Design review of the part built by this model. Coordinates are the model's own, in mm. Coordinates: 2 decimals unless noted, no trailing zeros. Order: outer loops, then holes, each group sorted by start corner. A loop starts at its lowest first (then second) coordinate and runs counter-clockwise, first axis right, second up. Notation, with made-up numbers: (11, -18) - (43, -18) arc R22 cw to (43, 15) - close; hole circle Ø2 at (66.5, 35). An arc over 180 degrees is marked (long way). Write each question's results on one line, items separated by ' | '. Start each with the question number.
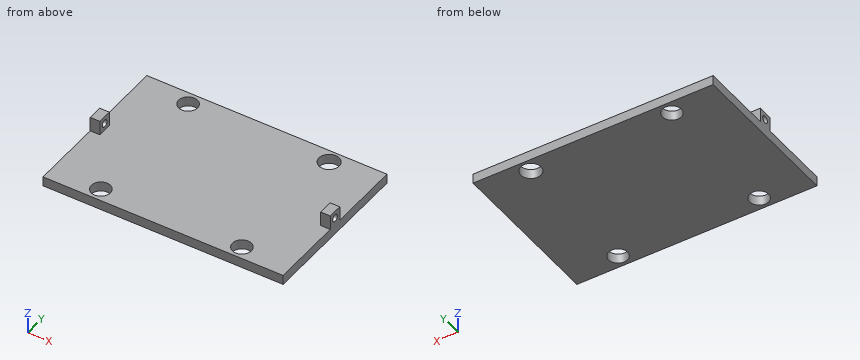
```python
from build123d import *

# Parameters (mm, degrees)
SKETCH1_W           = 49.5
SKETCH1_H           = 33
BOSS_EXTRUDE1_DEPTH = 2
BOSS_EXTRUDE4_DEPTH = 3
SKETCH9_R           = 0.75
CUT_EXTRUDE3_DEPTH  = 70
SKETCH10_R          = 2.087011894
SKETCH10_R_2        = 1.9558
CUT_EXTRUDE4_DEPTH  = 70


with BuildPart() as part:
    # Sketch1 → Boss-Extrude1 (new body)
    with BuildSketch(Plane.XY):
        with Locations((-6.974438903, -6.316084788)):
            Rectangle(SKETCH1_W, SKETCH1_H)
    extrude(amount=BOSS_EXTRUDE1_DEPTH)

    # Sketch8 → Boss-Extrude4 (add)
    with BuildSketch(Plane.XY.offset(2)):
        Polygon((-31.724438903, -6.316084788), (-31.724438903, -4.816084788), (-29.724438903, -4.816084788), (-29.724438903, -7.816084788), (-31.724438903, -7.816084788), align=None)
        Polygon((17.775561097, -4.816084788), (17.775561097, -7.816084788), (15.775561097, -7.816084788), (15.775561097, -6.316084788), (15.775561097, -4.816084788), align=None)
    extrude(amount=BOSS_EXTRUDE4_DEPTH)

    # Sketch9 → Cut-Extrude3 (cut)
    with BuildSketch(Plane.ZY.offset(31.724438903)):
        with Locations((3.5, -6.316084788)):
            Circle(SKETCH9_R)
    extrude(amount=-CUT_EXTRUDE3_DEPTH, mode=Mode.SUBTRACT)

    # Sketch10 → Cut-Extrude4 (cut)
    with BuildSketch(Plane(origin=(0, 0, 0), x_dir=(-1, 0, 0), z_dir=(0, 0, -1))):
        with Locations((-7.565561097, 7.539615212)):
            Circle(SKETCH10_R)
        with Locations((21.514438903, 7.539615212)):
            Circle(SKETCH10_R_2)
        with Locations((-7.565561097, -20.171784788)):
            Circle(SKETCH10_R_2)
        with Locations((21.514438903, -20.171784788)):
            Circle(SKETCH10_R_2)
    extrude(amount=-CUT_EXTRUDE4_DEPTH, mode=Mode.SUBTRACT)


solid = part.part
```
(1) Take a section at A-A (z = 3.5). State the section outline as (x, y) points, plus the area to 3 significant figures.
(2) Take a section at B-B (y = 8.5). State the section outline as (x, z) points.
(3) To check wall thickness, follow line 1 along Y through (x, z) = (16.35, 3.5); line 2 along X through (y, z) = (-7, 2.1); line 3 along X through (y, z) = (-21, 1.9). State the ranges of each line that lie inside material, in increasing order. Write a range as [from, to].
(4) Take a section at C-C (x = -13.5). State the section outline as (y, z) points.
(5) Take a section at D-D (y = 4.5). State the section outline as (x, z) points.
(6) Clearance check with flat-ended pins moving along their axes: pin 1 (1 mm diameter, centred on x = 16.5, z = 4, fed in from +Y); pin 2 (2.5 mm diameter, centred on x = -21.51, y = 7.54, fed in from +Z); pin 3 (1 mm diameter, centred on x = -25.5, y = -8.5, fed in from +Z); pin 4 (2 mm diameter, centred on x = -31, z = 3.5, fed in from -Y). State where each tip first meets the part, or that it passes through.
Worked out:
1) outline: (-31.72, -7.82) - (-29.72, -7.82) - (-29.72, -7.07) - (-31.72, -7.07) - close; (-31.72, -5.57) - (-29.72, -5.57) - (-29.72, -4.82) - (-31.72, -4.82) - close; (15.78, -7.82) - (17.78, -7.82) - (17.78, -7.07) - (15.78, -7.07) - close; (15.78, -5.57) - (17.78, -5.57) - (17.78, -4.82) - (15.78, -4.82) - close | area: 6.00 mm^2
2) outline: (-31.72, 0) - (-23.22, 0) - (-23.22, 2) - (-31.72, 2) - close; (-19.81, 0) - (5.71, 0) - (5.71, 2) - (-19.81, 2) - close; (9.42, 0) - (17.78, 0) - (17.78, 2) - (9.42, 2) - close
3) line 1: [-7.82, -7.07], [-5.57, -4.82] | line 2: [-31.72, -29.72], [15.78, 17.78] | line 3: [-31.72, -23.29], [-19.74, 5.79], [9.34, 17.78]
4) outline: (-22.82, 0) - (10.18, 0) - (10.18, 2) - (-22.82, 2) - close
5) outline: (-31.72, 0) - (17.78, 0) - (17.78, 2) - (-31.72, 2) - close
6) pin 1: y = -4.82 | pin 2: through | pin 3: z = 2 | pin 4: y = -7.82
